Source: CAD feature listing. Evaluate the final solid. Frame: model axes, mm. Give positions to 0.01 mm unless a question says otherwise; leave off trailing zeros. Write each loop counter-clockwise with the first axis right and the second up, starting at its lowest first coordinate (ties: lowest second). Pieces come first, ordered by that corner, then holes.
```python
from build123d import *

# Parameters (mm, degrees)
PAD_DEPTH     = 2.032
SKETCH002_W   = 12.7
SKETCH002_H   = 10.16
SKETCH002_H_2 = 15.24
POCKET_DEPTH  = 5.0038


with BuildPart() as part:
    # Sketch → Pad (new body)
    with BuildSketch(Plane.XY):
        with BuildLine():
            ThreePointArc((-93.98, 48.26), (-102.062231, 44.912231), (-105.41, 36.83))
            Line((-105.41, -36.83), (-105.41, 36.83))
            ThreePointArc((-105.41, -36.83), (-102.062231, -44.912231), (-93.98, -48.26))
            Line((93.98, -48.26), (-93.98, -48.26))
            ThreePointArc((93.98, -48.26), (102.062231, -44.912231), (105.41, -36.83))
            Line((105.41, 36.83), (105.41, -36.83))
            ThreePointArc((105.41, 36.83), (102.062231, 44.912231), (93.98, 48.26))
            Line((-93.98, 48.26), (93.98, 48.26))
        make_face()
    extrude(amount=PAD_DEPTH)

    # Sketch002 (on Face9 of Pad) → Pocket (cut)
    with BuildSketch(Plane(origin=(0, 0, 0), x_dir=(1, 0, 0), z_dir=(0, 0, -1))):
        with BuildLine():
            ThreePointArc((-83.82, 39.37), (-85.616051, 38.626051), (-86.36, 36.83))
            Line((-86.36, -36.83), (-86.36, 36.83))
            ThreePointArc((-86.36, -36.83), (-85.616051, -38.626051), (-83.82, -39.37))
            Line((83.82, -39.37), (-83.82, -39.37))
            ThreePointArc((83.82, -39.37), (85.616051, -38.626051), (86.36, -36.83))
            Line((86.36, 36.83), (86.36, -36.83))
            ThreePointArc((86.36, 36.83), (85.616051, 38.626051), (83.82, 39.37))
            Line((-83.82, 39.37), (83.82, 39.37))
        make_face()
        with Locations((-99.06, 0)):
            Rectangle(SKETCH002_W, SKETCH002_H)
        with Locations((-99.06, -26.67)):
            Rectangle(SKETCH002_W, SKETCH002_H_2)
    extrude(amount=-POCKET_DEPTH, mode=Mode.SUBTRACT)


solid = part.part
```
1. Contact query for flat-ended pins moving along their axis: P1, Ø1, axis at y = 0, z = 1, coming from the -X side; P2, Ø0.6, axis at x = -97.5, z = 1, coming from the -Y side. Output: stop coordinate, or through.
2. Cut plane A-A, the plane y = -7.5. Return the cut outline in (x, z), then the cut area to 3 significant figures.
3. Cut plane C-C, the plane x = -79. Return the cut outline in (y, z).
4. Cut plane B-B, the plane z = 1.05. Return the cut outline in (x, y).
5. Line query: L1, parallel to X at y = -2, z = 0.9; L2, parallel to Y at x = -50.5, z = 0.65; L3, parallel to X at y = -14, z = 1.1. Output: solid intervals per line, ascending.
Response values:
1. P1: stops at x = -92.71
1. P2: stops at y = -47.8
2. outline: (-105.41, 0) - (-86.36, 0) - (-86.36, 2.03) - (-105.41, 2.03) - close; (86.36, 0) - (105.41, 0) - (105.41, 2.03) - (86.36, 2.03) - close
2. area: 77.4 mm2
3. outline: (-48.26, 0) - (-39.37, 0) - (-39.37, 2.03) - (-48.26, 2.03) - close; (39.37, 0) - (48.26, 0) - (48.26, 2.03) - (39.37, 2.03) - close
4. outline: (-105.41, -36.83) arc R11.43 ccw to (-93.98, -48.26) - (93.98, -48.26) arc R11.43 ccw to (105.41, -36.83) - (105.41, 36.83) arc R11.43 ccw to (93.98, 48.26) - (-93.98, 48.26) arc R11.43 ccw to (-105.41, 36.83) - (-105.41, 34.29) - (-92.71, 34.29) - (-92.71, 19.05) - (-105.41, 19.05) - (-105.41, 5.08) - (-92.71, 5.08) - (-92.71, -5.08) - (-105.41, -5.08) - close; hole (-86.36, -36.83) arc R2.54 ccw to (-83.82, -39.37) - (83.82, -39.37) arc R2.54 ccw to (86.36, -36.83) - (86.36, 36.83) arc R2.54 ccw to (83.82, 39.37) - (-83.82, 39.37) arc R2.54 ccw to (-86.36, 36.83) - close
5. L1: x = -92.71 to -86.36, 86.36 to 105.41
5. L2: y = -48.26 to -39.37, 39.37 to 48.26
5. L3: x = -105.41 to -86.36, 86.36 to 105.41
